from build123d import *

# Parameters (mm, degrees)
BOSS_EXTRUDE1_DEPTH = 2
BOSS_EXTRUDE2_DEPTH = 5
SKETCH3_W           = 0.8
SKETCH3_H           = 1.5
CUT_EXTRUDE1_DEPTH  = 5
SKETCH4_W           = 4.8
SKETCH4_H           = 1.5
BOSS_EXTRUDE3_DEPTH = 1
CHAMFER3_SIZE       = 0.6
CHAMFER3_SIZE_2     = 1.286704152
SKETCH6_W           = 2.6
SKETCH6_H           = 10.9
CUT_EXTRUDE2_DEPTH  = 49.169310769
SKETCH7_W           = 5.6
SKETCH7_H           = 13.9
SKETCH7_W_2         = 2.6
SKETCH7_H_2         = 10.9
BOSS_EXTRUDE4_DEPTH = 6.5
CHAMFER6_SIZE       = 0.5
FILLET1_R           = 4


with BuildPart() as part:
    # Sketch1 → Boss-Extrude1 (new body)
    with BuildSketch(Plane(origin=(0, 0, 0), x_dir=(1, 0, 0), z_dir=(0, 1, 0))):
        Polygon((-42.35, 10.5), (-29.75, 10.5), (-29.75, -10.5), (-42.35, -10.5), (-42.35, -22.4), (42.35, -22.4), (42.35, 22.4), (-42.35, 22.4), align=None)
    extrude(amount=BOSS_EXTRUDE1_DEPTH)

    # Sketch2 → Boss-Extrude2 (add)
    with BuildSketch(Plane(origin=(0, 2, 0), x_dir=(1, 0, 0), z_dir=(0, 1, 0))):
        Polygon((-40.35, 20.4), (-40.35, 10.5), (-29.75, 10.5), (-29.75, -10.5), (-40.35, -10.5), (-40.35, -20.4), (40.35, -20.4), (40.35, 20.4), align=None)
        Polygon((-38.85, -12), (-38.85, -18.9), (38.85, -18.9), (38.85, 18.9), (-38.85, 18.9), (-38.85, 12), (-28.25, 12), (-28.25, -12), align=None, mode=Mode.SUBTRACT)
    extrude(amount=BOSS_EXTRUDE2_DEPTH)

    # Sketch3 → Cut-Extrude1 (cut)
    with BuildSketch(Plane(origin=(0, 7, 0), x_dir=(1, 0, 0), z_dir=(0, 1, 0))):
        with Locations((-25.15, 19.65)):
            Rectangle(SKETCH3_W, SKETCH3_H)
        with Locations((-19.55, 19.65)):
            Rectangle(SKETCH3_W, SKETCH3_H)
        with Locations((-19.55, -19.65)):
            Rectangle(SKETCH3_W, SKETCH3_H)
        with Locations((-25.15, -19.65)):
            Rectangle(SKETCH3_W, SKETCH3_H)
        with Locations((19.55, 19.65)):
            Rectangle(SKETCH3_W, SKETCH3_H)
        with Locations((25.15, 19.65)):
            Rectangle(SKETCH3_W, SKETCH3_H)
        with Locations((25.15, -19.65)):
            Rectangle(SKETCH3_W, SKETCH3_H)
        with Locations((19.55, -19.65)):
            Rectangle(SKETCH3_W, SKETCH3_H)
    extrude(amount=-CUT_EXTRUDE1_DEPTH, mode=Mode.SUBTRACT)

    # Sketch4 → Boss-Extrude3 (add)
    with BuildSketch(Plane.XY.offset(20.4)):
        with Locations((-22.35, 6.25)):
            Rectangle(SKETCH4_W, SKETCH4_H)
        with Locations((22.35, 6.25)):
            Rectangle(SKETCH4_W, SKETCH4_H)
    boss_extrude3 = extrude(amount=BOSS_EXTRUDE3_DEPTH)

    # Mirror1: Boss-Extrude3 across plane
    add(boss_extrude3.mirror(Plane.XY))

    # Chamfer3
    # the kernel refuses this chamfer: 1.286704152, 0.6 mm, written as the material it takes off along each edge
    with BuildSketch(Plane(origin=(16.616181102, 5.5, -21.4), x_dir=(0, 0.9971975577536771, -0.07481330637060246), z_dir=(1, 0, 0))) as chamfer3_piece_1_section:
        Polygon((CHAMFER3_SIZE * 0.997197557754, CHAMFER3_SIZE * 0.0748133063706), (-CHAMFER3_SIZE_2 * 0.0748133063884, CHAMFER3_SIZE_2 * 0.997197557991), (0, 0), align=None)
    chamfer3_piece_1 = extrude(amount=11.467637795, mode=Mode.PRIVATE)
    chamfer3_piece_1 = split(chamfer3_piece_1, bisect_by=Plane(origin=(22.35, 5.708120407, -20.4), z_dir=(0, 0, -1)), keep=Keep.TOP, mode=Mode.PRIVATE)
    add(chamfer3_piece_1, mode=Mode.SUBTRACT)
    with BuildSketch(Plane(origin=(28.083818898, 7, -21.4), x_dir=(0, 0.016311164131109942, 0.9998669641130704), z_dir=(-1, 0, 0))) as chamfer3_piece_2_section:
        Polygon((CHAMFER3_SIZE_2 * 0.999866964351, -CHAMFER3_SIZE_2 * 0.016311164135), (-CHAMFER3_SIZE * 0.0163111641311, -CHAMFER3_SIZE * 0.999866964113), (0, 0), align=None)
    chamfer3_piece_2 = extrude(amount=8.133818898, mode=Mode.PRIVATE)
    chamfer3_piece_2 = split(chamfer3_piece_2, bisect_by=Plane(origin=(25.55, 6.955435886, -20.304431949), z_dir=(-1, 0, 0)), keep=Keep.TOP, mode=Mode.PRIVATE)
    add(chamfer3_piece_2, mode=Mode.SUBTRACT)
    with BuildSketch(Plane(origin=(-16.616181102, 5.5, -21.4), x_dir=(0, 0.9971975577536771, -0.07481330637060246), z_dir=(-1, 0, 0))) as chamfer3_piece_3_section:
        Polygon((CHAMFER3_SIZE * 0.997197557754, -CHAMFER3_SIZE * 0.0748133063706), (-CHAMFER3_SIZE_2 * 0.0748133063884, -CHAMFER3_SIZE_2 * 0.997197557991), (0, 0), align=None)
    chamfer3_piece_3 = extrude(amount=11.467637795, mode=Mode.PRIVATE)
    chamfer3_piece_3 = split(chamfer3_piece_3, bisect_by=Plane(origin=(-22.35, 5.708120407, -20.4), z_dir=(0, 0, -1)), keep=Keep.TOP, mode=Mode.PRIVATE)
    add(chamfer3_piece_3, mode=Mode.SUBTRACT)
    with BuildSketch(Plane(origin=(-24.75, 7, -21.4), x_dir=(0, 0.016311164131109942, 0.9998669641130704), z_dir=(1, 0, 0))) as chamfer3_piece_4_section:
        Polygon((CHAMFER3_SIZE_2 * 0.999866964351, CHAMFER3_SIZE_2 * 0.016311164135), (-CHAMFER3_SIZE * 0.0163111641311, CHAMFER3_SIZE * 0.999866964113), (0, 0), align=None)
    chamfer3_piece_4 = extrude(amount=8.133818898, mode=Mode.PRIVATE)
    chamfer3_piece_4 = split(chamfer3_piece_4, bisect_by=Plane(origin=(-19.15, 6.955435886, -20.304431949), z_dir=(-1, 0, 0)), keep=Keep.TOP, mode=Mode.PRIVATE)
    add(chamfer3_piece_4, mode=Mode.SUBTRACT)
    with BuildSketch(Plane(origin=(16.616181102, 5.5, 21.4), x_dir=(0, 0.9971975577536771, 0.07481330637060246), z_dir=(1, 0, 0))) as chamfer3_piece_5_section:
        Polygon((CHAMFER3_SIZE * 0.997197557754, -CHAMFER3_SIZE * 0.0748133063706), (-CHAMFER3_SIZE_2 * 0.0748133063884, -CHAMFER3_SIZE_2 * 0.997197557991), (0, 0), align=None)
    chamfer3_piece_5 = extrude(amount=11.467637795, mode=Mode.PRIVATE)
    chamfer3_piece_5 = split(chamfer3_piece_5, bisect_by=Plane(origin=(22.35, 5.708120407, 20.4), z_dir=(0, 0, 1)), keep=Keep.TOP, mode=Mode.PRIVATE)
    add(chamfer3_piece_5, mode=Mode.SUBTRACT)
    with BuildSketch(Plane(origin=(24.75, 7, 21.4), x_dir=(0, 0.016311164131109942, -0.9998669641130704), z_dir=(-1, 0, 0))) as chamfer3_piece_6_section:
        Polygon((CHAMFER3_SIZE_2 * 0.999866964351, CHAMFER3_SIZE_2 * 0.016311164135), (-CHAMFER3_SIZE * 0.0163111641311, CHAMFER3_SIZE * 0.999866964113), (0, 0), align=None)
    chamfer3_piece_6 = extrude(amount=8.133818898, mode=Mode.PRIVATE)
    chamfer3_piece_6 = split(chamfer3_piece_6, bisect_by=Plane(origin=(19.15, 6.955435886, 20.304431949), z_dir=(1, 0, 0)), keep=Keep.TOP, mode=Mode.PRIVATE)
    add(chamfer3_piece_6, mode=Mode.SUBTRACT)
    with BuildSketch(Plane(origin=(-24.75, 7, 21.4), x_dir=(0, 0.016311164131109942, -0.9998669641130704), z_dir=(1, 0, 0))) as chamfer3_piece_7:
        Polygon((CHAMFER3_SIZE_2 * 0.999866964351, -CHAMFER3_SIZE_2 * 0.016311164135), (-CHAMFER3_SIZE * 0.0163111641311, -CHAMFER3_SIZE * 0.999866964113), (0, 0), align=None)
    extrude(amount=4.8, mode=Mode.SUBTRACT)
    with BuildSketch(Plane(origin=(-16.616181102, 5.5, 21.4), x_dir=(0, 0.9971975577536771, 0.07481330637060246), z_dir=(-1, 0, 0))) as chamfer3_piece_8_section:
        Polygon((CHAMFER3_SIZE * 0.997197557754, CHAMFER3_SIZE * 0.0748133063706), (-CHAMFER3_SIZE_2 * 0.0748133063884, CHAMFER3_SIZE_2 * 0.997197557991), (0, 0), align=None)
    chamfer3_piece_8 = extrude(amount=11.467637795, mode=Mode.PRIVATE)
    chamfer3_piece_8 = split(chamfer3_piece_8, bisect_by=Plane(origin=(-22.35, 5.708120407, 20.4), z_dir=(0, 0, 1)), keep=Keep.TOP, mode=Mode.PRIVATE)
    add(chamfer3_piece_8, mode=Mode.SUBTRACT)

    # Sketch6 → Cut-Extrude2 (cut, through all)
    with BuildSketch(Plane(origin=(0, 2, 0), x_dir=(1, 0, 0), z_dir=(0, 1, 0))):
        with Locations((33.55, 0)):
            Rectangle(SKETCH6_W, SKETCH6_H)
    extrude(amount=-CUT_EXTRUDE2_DEPTH, mode=Mode.SUBTRACT)

    # Sketch7 → Boss-Extrude4 (add)
    with BuildSketch(Plane(origin=(0, 2, 0), x_dir=(1, 0, 0), z_dir=(0, 1, 0))):
        with Locations((33.55, 0)):
            Rectangle(SKETCH7_W, SKETCH7_H)
        with Locations((33.55, 0)):
            Rectangle(SKETCH7_W_2, SKETCH7_H_2, mode=Mode.SUBTRACT)
    extrude(amount=BOSS_EXTRUDE4_DEPTH)

    # Chamfer6
    chamfer6_edges = [part.edges().sort_by_distance(p)[0] for p in [
        (-36.05, 0, -10.5),
        (-42.35, 0, -16.45),
        (0, 0, -22.4),
        (42.35, 0, 0),
        (0, 0, 22.4),
        (-42.35, 0, 16.45),
        (-36.05, 0, 10.5),
        (-29.75, 0, 0),
    ]]
    chamfer(chamfer6_edges, length=CHAMFER6_SIZE)

    # Fillet1
    fillet1_edges = [part.edges().sort_by_distance(p)[0] for p in [
        (-22.35, 2, 18.9),
        (22.35, 2, 18.9),
        (22.35, 2, -18.9),
        (-22.35, 2, -18.9),
    ]]
    fillet(fillet1_edges, radius=FILLET1_R)


solid = part.part
Could you check a few things on this model? Use its own coordinates, in mm. A direction names the side the tool comes from. Coordinates: 2 decimals unless noted, no trailing zeros. Loops run counter-clockwise (first coordinate to the right, second up) from the corner with the lowest first, then second, coordinate; pieces in that order, holes last.
1. I need wall thicknesses on L1, parallel to X at y = 4, z = -1; L2, parallel to Z at x = 35, y = 4; L3, parallel to Z at x = -32, y = 3. Which ranges of each line are inside material? Lowest first, please.
2. Imagine slicing it at D-D (y = 4). Give the number of separate pieces and of enclosed holes in the cut face, and give its area (3 significant figures).
3. For faces 1 (the face through (40.35, 4, 0)), 2 (the face through (-33, 4, -20.4)), 3 (the face through (-33, 4, 20.4)), 4 (the face through (-40.35, 4, 15)), which set-ups out of +Z, -Z, +X, -X, +Y, -Y let a thin tool reach every point of the face, with its end or its side?
4. For P1, Ø1.5, axis at x = -35.5, y = 4.5, coming from the +Z side; P2, Ø4, axis at x = -29.5, y = 7, coming from the -Z side; P3, Ø6, axis at x = 15.5, z = -10, coming from the +Y side; P4, Ø1.5, axis at x = -31.5, z = 1, coming from the -Y side, each with a flat end and sliding along its axis, tell me the tip position at first contact or that it passes through.
5. Imagine slicing it at B-B (z = 1.5). Please give me the cut outline in (x, y).
6. Imagine slicing it at C-C (x = -16.5). Please give me the cut outline in (y, z), and give its area (3 significant figures).
7. Imagine slicing it at A-A (x = -34.5). Please give me the cut outline in (y, z), and give its area (3 significant figures).
8. We'd pull the mould along Z, two halves only. Please class faces 5 (the face through (34, 4, -5.45)), 6 (the face through (22, 4, 20.4)), 7 (the face through (-25.55, 5, 20)): released by +Z, released by -Z, zero draft, split by the parting line, or undercut.
Computed values:
1. L1: x = -29.75 to -28.25, 30.75 to 32.25, 34.85 to 36.35, 38.85 to 40.35
1. L2: z = -20.4 to -18.9, -6.95 to 6.95, 18.9 to 20.4
1. L3: z = -20.4 to -18.9, -12 to -10.5, 10.5 to 12, 18.9 to 20.4
2. separate pieces: 9
2. enclosed holes: 1
2. area: 437 mm2
3. face 1: +Z, -Z, +X, +Y
3. face 2: -Z, -X, +Y
3. face 3: +Z, -X, +Y
3. face 4: +Z, -Z, -X, +Y
4. P1: stops at z = 20.4
4. P2: stops at z = -20.4
4. P3: stops at y = 2
4. P4: passes through
5. outline: (-29.75, 0.5) - (-29.25, 0) - (32.25, 0) - (32.25, 8.5) - (30.75, 8.5) - (30.75, 2) - (-28.25, 2) - (-28.25, 7) - (-29.75, 7) - close; (34.85, 0) - (41.85, 0) - (42.35, 0.5) - (42.35, 2) - (40.35, 2) - (40.35, 7) - (38.85, 7) - (38.85, 2) - (36.35, 2) - (36.35, 8.5) - (34.85, 8.5) - close
6. outline: (0, -21.9) - (0.5, -22.4) - (2, -22.4) - (2, -20.4) - (7, -20.4) - (7, -18.9) - (2, -18.9) - (2, 18.9) - (7, 18.9) - (7, 20.4) - (2, 20.4) - (2, 22.4) - (0.5, 22.4) - (0, 21.9) - close
6. area: 104 mm2
7. outline: (0, -21.9) - (0.5, -22.4) - (2, -22.4) - (2, -20.4) - (7, -20.4) - (7, -18.9) - (2, -18.9) - (2, -12) - (7, -12) - (7, -10.5) - (0.5, -10.5) - (0, -11) - close; (0, 11) - (0.5, 10.5) - (7, 10.5) - (7, 12) - (2, 12) - (2, 18.9) - (7, 18.9) - (7, 20.4) - (2, 20.4) - (2, 22.4) - (0.5, 22.4) - (0, 21.9) - close
7. area: 77.1 mm2
8. face 5: undercut
8. face 6: released by +Z
8. face 7: zero draft
